Design review of the part built by this model. Coordinates are the model's own, in mm. Coordinates: 2 decimals unless noted, no trailing zeros. Order: outer loops, then holes, each group sorted by start corner. A loop starts at its lowest first (then second) coordinate and runs counter-clockwise, first axis right, second up. Notation, with made-up numbers: M 67,65 L 104,65 A19 cw 104,85 Z; hole C -36.75,-15 d7. An arc over 180 degrees is marked long. Answer as a JSON object with one key per item and string values.
from build123d import *

# Parameters (mm, degrees)
SKETCH1_R           = 10
BOSS_EXTRUDE1_DEPTH = 10


with BuildPart() as part:
    # Sketch1 → Boss-Extrude1 (new body)
    with BuildSketch(Plane.XY):
        with BuildLine():
            Line((-15, -75.267843328), (-10, -75.267843328))
            ThreePointArc((-10, -75.267843328), (0, -65.267843328), (10, -75.267843328))
            Line((10, -75.267843328), (15, -75.267843328))
            Line((15, -75.267843328), (20, -75.267843328))
            Line((20, -75.267843328), (20, -63.153600369))
            Line((20, -63.153600369), (14.459340055, -63.153600369))
            add(Edge.make_bspline(
                [(15, 204.732156672), (8.134301698, 174.35100944), (7.954081716, 85.055757093), (14.459340055, -63.153600369)],
                knots=[0, 0, 0, 0, 0.97375067, 0.97375067, 0.97375067, 0.97375067], degree=3))
            ThreePointArc((15, 204.732156672), (0, 219.732156672), (-15, 204.732156672))
            add(Edge.make_bspline(
                [(-15, 204.732156672), (-9.431523273, 174.705672452), (-9.285696116, 85.410420106), (-14.56251853, -63.153600369)],
                knots=[0, 0, 0, 0, 0.97381202, 0.97381202, 0.97381202, 0.97381202], degree=3))
            Line((-14.56251853, -63.153600369), (-20, -63.153600369))
            Line((-20, -63.153600369), (-20, -75.267843328))
            Line((-20, -75.267843328), (-15, -75.267843328))
        make_face()
        with Locations((0, 204.732156672)):
            Circle(SKETCH1_R, mode=Mode.SUBTRACT)
    extrude(amount=BOSS_EXTRUDE1_DEPTH)

    # Sketch7 → Ø4.0 (4) Diameter Hole2 (revolve, cut)
    with BuildSketch(Plane(origin=(-17, -75.267843328, 5), x_dir=(0, 0, -1), z_dir=(1, 0, 0))):
        Polygon((0, 0), (0, 11.201721238), (2, 10), (2, 0), align=None)
    f_4_0_4_diameter_hole2 = revolve(axis=Axis((-17, -81.617843328, 5), (0, 1, 0)), mode=Mode.SUBTRACT)

    # Mirror2: Ø4.0 (4) Diameter Hole2 across plane
    add(f_4_0_4_diameter_hole2.mirror(Plane(origin=(0, 0, 0), x_dir=(0, 0, 1), z_dir=(1, 0, 0))), mode=Mode.SUBTRACT)


solid = part.part
1) Add section A-A (x = 5). State the section outline as (y, z) points.
Taken from the geometry:
{"outline": "M -66.61,0 L 196.07,0 L 196.07,10 L -66.61,10 Z; M 213.39,0 L 218.87,0 L 218.87,10 L 213.39,10 Z"}
2) To check wall thickness, follow L1, parallel to Y at x = 0, z = 3.25; L2, parallel to Z at x = -17, y = -70; L3, parallel to X at y = -69.5, z = 5. State the ranges of each line that lie inside material, in increasing order.
Taken from the geometry:
{"L1": "y = -65.27 to 194.73, 214.73 to 219.73", "L2": "z = 0 to 3, 7 to 10", "L3": "x = -20 to -19, -15 to -8.17, 8.17 to 15, 19 to 20"}
3) Insertion check: pin 1 Ø2 at (x, z) = (4.5, 6.5) entering from -Y; pin 2 Ø1.6 at (x, z) = (-18, 6.5) entering from +Y; pin 3 Ø4 at (x, y) = (-10, 76) entering from -Z; pin 4 Ø6 at (y, z) = (181, 5.5) entering from -X. Each pin has a flat end and moves straight along its axis. Give the tip position at first contact, or say it passes through.
Taken from the geometry:
{"pin 1": "stops at y = -66.92", "pin 2": "stops at y = -63.15", "pin 3": "stops at z = 0", "pin 4": "stops at x = -12.61"}
4) Mouldability with a two-part tool opening along X and no side actions: class faces 1 (the cylindrical face through (-2.17, 194.97, 4.93)), 2 (the cylindrical face through (0.33, 219.73, 4.93)), 3 (the flat face through (-14, -75.268, 5)) as released by +X, released by -X, zero draft, split by the parting line, or undercut.
Taken from the geometry:
{"face 1": "undercut", "face 2": "split by the parting line", "face 3": "zero draft"}
